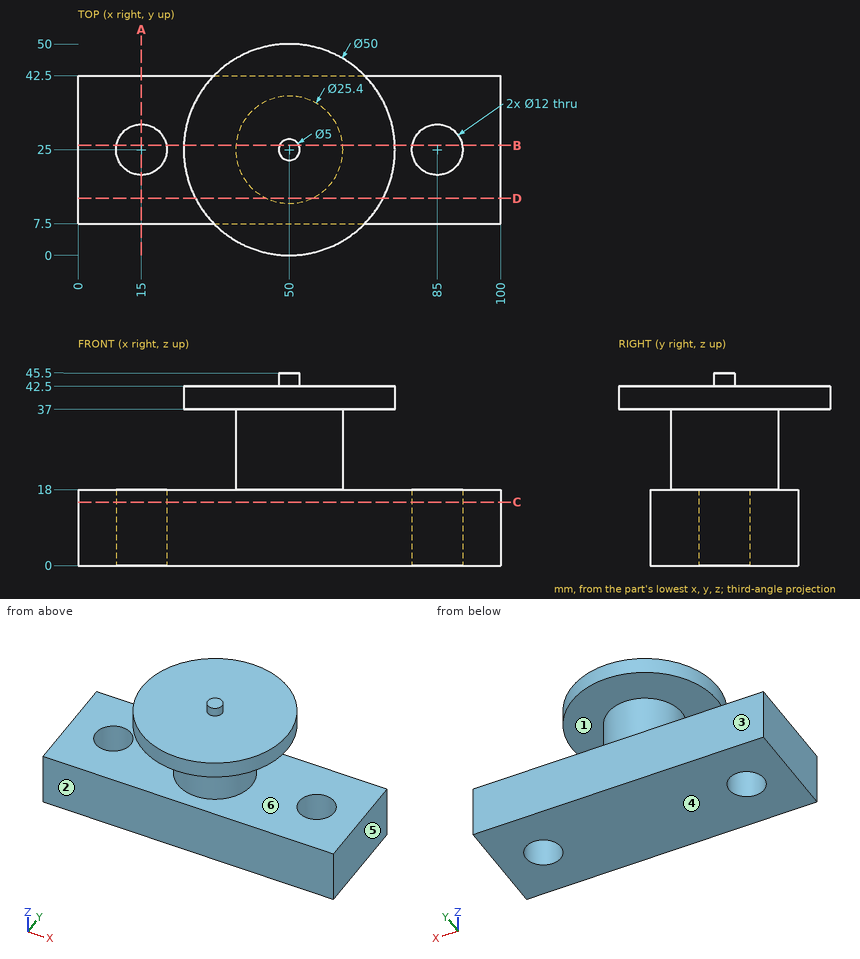
The figure shows three views and two pictorial views of one solid part (mm, origin at its lowest corner). Answer the questions. A direction names the side the tool comes from. Coordinates: 2 decimals unless noted, no trailing zeros. Write each loop counter-clockwise with the first axis right and the second up, starting at its lowest first coordinate (ties: lowest second). Pieces come first, ordered by that corner, then holes. Notation, with made-up numbers: M 89,-13.75 L 105,-13.75 A25 cw 105,11.25 Z; hole C 9,8.25 d1. An arc over 180 degrees is marked long. Answer as CSV lines item,"result". Start each with the question number.
Item 1: Section A-A on x = 15 is taken. Write down the section's boundary in (y, z).
Item 2: Determine the mould class of the marked faces 4, 5 and 6 for opening direction Z: released by +Z, released by -Z, zero draft, split by the parting line, or undercut.
Item 3: Consider L1, parallel to Y at x = 85, z = 12; L2, parallel to Y at x = 5, z = 13.5; L3, parallel to X at y = 26.5, z = 14. Determine where each line is inside the solid, lowest interval first.
Item 4: Section D-D on y = 13.5 is taken. Write down the section's boundary in (x, z).
Item 5: Section B-B on y = 26 is taken. Write down the section's boundary in (x, z), and give its area (3 significant figures).
Item 6: Flat-ended cylindrical pins translate along their axes: P1, Ø1, axis at x = 83.5, y = 42, coming from the +Z side; P2, Ø3, axis at x = 84.5, z = 17.5, coming from the -Y side; P3, Ø6, axis at x = 47, z = 36.5, coming from the +Y side; P4, Ø12, axis at x = 26.5, z = 28.5, coming from the -Y side. Find the tip coordinate at first contact, or state that the pin passes through.
Item 7: A tool of negligible diameter and unlimited length cuts with its end or side. For the marked faces 1, 2 and 3, from which of +Z, -Z, +X, -X, +Y, -Y can it reach the whole face along a straight path? Write none if from no direction.
Item 8: Section C-C on z = 15 is taken. Write down the section's boundary in (x, y).
Checks:
1,outline,"M 7.5,0 L 19,0 L 19,18 L 7.5,18 Z; M 31,0 L 42.5,0 L 42.5,18 L 31,18 Z"
2,face 4,"released by -Z"
2,face 5,"zero draft"
2,face 6,"undercut"
3,L1,"y = 7.5 to 19, 31 to 42.5"
3,L2,"y = 7.5 to 42.5"
3,L3,"x = 0 to 9.19, 20.81 to 79.19, 90.81 to 100"
4,outline,"M 0,0 L 100,0 L 100,18 L 55.39,18 L 55.39,37 L 72.2,37 L 72.2,42.5 L 27.8,42.5 L 27.8,37 L 44.61,37 L 44.61,18 L 0,18 Z"
5,outline,"M 0,0 L 9.08,0 L 9.08,18 L 0,18 Z; M 20.92,0 L 79.08,0 L 79.08,18 L 62.66,18 L 62.66,37 L 74.98,37 L 74.98,42.5 L 52.29,42.5 L 52.29,45.5 L 47.71,45.5 L 47.71,42.5 L 25.02,42.5 L 25.02,37 L 37.34,37 L 37.34,18 L 20.92,18 Z; M 90.92,0 L 100,0 L 100,18 L 90.92,18 Z"
5,area,"2,140 mm²"
6,P1,"stops at z = 18"
6,P2,"stops at y = 7.5"
6,P3,"stops at y = 50"
6,P4,"passes through"
7,face 1,"none"
7,face 2,"-Z, +X, -X, -Y"
7,face 3,"-Z, +X, -X, +Y"
8,outline,"M 0,7.5 L 100,7.5 L 100,42.5 L 0,42.5 Z; hole C 15,25 d12; hole C 85,25 d12"
